Drawing for the job (mm, zero at the part's lowest x, y, z). A direction names the side the tool comes from. Give positions to 0.01 mm unless a question says otherwise; leave off trailing zeros. Loops run counter-clockwise (first coordinate to the right, second up) from the corner with the lowest first, then second, coordinate; pieces in that order, holes last. Notation, with made-up numbers: M -2.75,3.25 L 24.25,3.25 A18 ccw 24.25,27.25 Z; hole C 29.25,57.5 d5. An arc over 180 degrees is marked long. Use CSV: the item, a comma, the result in double quotes. Start each with the question number.
(1) Slice it at A-A on z = 5.75. List the corners of the cut face in (x, y).
(2) Slice it at B-B on y = 21. List the corners of the cut face in (x, z), and give its area (3 significant figures).
(3) Tool access for the marked faces 1, 2, 3 and 4: list every direction of +Z, -Z, +X, -X, +Y, -Y with a clear straight run to the whole face (end or side of a thin tool).
(4) Flat gauge pins, fed straight in: P1, Ø2.5, axis at y = 4, z = 6, coming from the +X side; P2, Ø5, axis at y = 37.5, z = 2, coming from the -X side; P3, Ø4.5, axis at y = 14.5, z = 5, coming from the -X side; P4, Ø4.5, axis at x = 3.5, z = 5.5, coming from the +Y side. Where does each tip first touch, or does it go through?
(5) Wall check: line 1 along Y through (x, z) = (49, 6.5); line 2 along X through (y, z) = (16, 7.75). Give the ranges that are in metal, low to high. Write a range as from..to.
(6) Slice it at C-C on x = 113. List the corners of the cut face in (y, z).
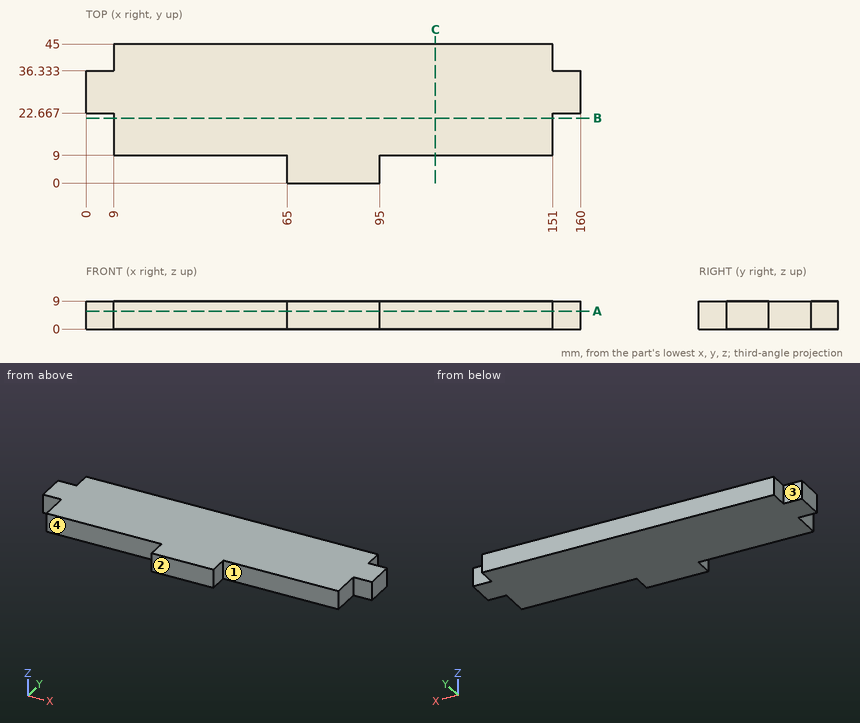
Reply:
1,outline,"M 0,22.67 L 9,22.67 L 9,9 L 65,9 L 65,0 L 95,0 L 95,9 L 151,9 L 151,22.67 L 160,22.67 L 160,36.33 L 151,36.33 L 151,45 L 9,45 L 9,36.33 L 0,36.33 Z"
2,outline,"M 9,0 L 151,0 L 151,9 L 9,9 Z"
2,area,"1,280 mm^2"
3,face 1,"+Z, -Z, +X, -Y"
3,face 2,"+Z, -Z, +X, -X, -Y"
3,face 3,"+Z, -Z, -X, +Y"
3,face 4,"+Z, -Z, -X, -Y"
4,P1,"stops at x = 95"
4,P2,"stops at x = 0"
4,P3,"stops at x = 9"
4,P4,"stops at y = 36.33"
5,line 1,"y = 9..45"
5,line 2,"x = 9..151"
6,outline,"M 9,0 L 45,0 L 45,9 L 9,9 Z"
